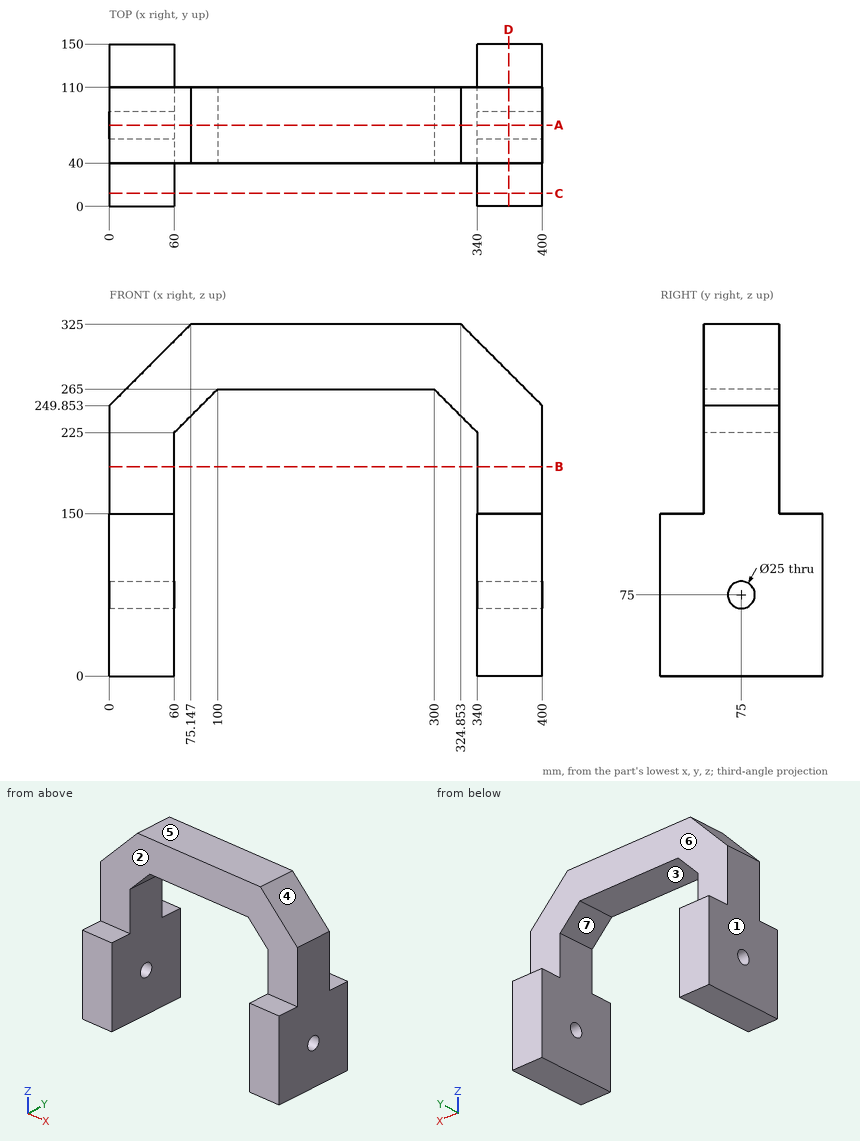
Here's the drawing with two shaded views (mm, measured from the low corner). I have some questions. A direction names the side the tool comes from. Coordinates: 2 decimals unless noted, no trailing zeros. Write each loop counter-clockwise with the first axis right and the second up, starting at its lowest first coordinate (ties: lowest second). Pieces come first, ordered by that corner, then holes. Notation, with made-up numbers: (17.5, 13.5) -> (22.5, 13.5) arc R36 ccw to (22.5, 52.5) -> close; hole circle Ø11 at (46.25, 13). An arc over 180 degrees is marked (long way). Write item = value, one per line. Start each with the question number.
(1) I want a section at B-B (z = 193.5). Please give me the cut outline in (x, y), plus the area to 3 significant figures.
(2) Which directions (+Z, -Z, +X, -X, +Y, -Y) give clear straight access to the entire face, cutting with the end or side of a thin tool? Please do the marked faces 5, 6 and 7.
(3) I want a section at C-C (y = 12). Please give me the cut outline in (x, z), plus the area to 3 significant figures.
(4) We'd pull the mould along X, two halves only. Please class the marked faces 1, 2, 3 and 4: released by +X, released by -X, zero draft, split by the parting line, or undercut.
(5) I want a section at A-A (y = 75). Please give me the cut outline in (x, z).
(6) Will these pins go through, and if not, where does the flat tip stop? pin 1 (12 mm diameter, centred on x = 18.5, y = 24, fed in from +Z); pin 2 (5 mm diameter, centred on x = 80.5, y = 76, fed in from -Z); pin 3 (12 mm diameter, centred on x = 199, y = 100, fed in from -Z).
(7) I need wall thicknesses on line 1 (X direction, y = 17, z = 122); line 2 (Y direction, x = 31, z = 245); line 3 (Z direction, x = 361, y = 111). Which ranges of each line are inside material? Lowest first, please. Write a range as [from, to].
(8) I want a section at D-D (x = 369). Please give me the cut outline in (y, z), plus the area to 3 significant figures.
Result set:
q1.outline = (0, 40) -> (60, 40) -> (60, 110) -> (0, 110) -> close; (340, 40) -> (400, 40) -> (400, 110) -> (340, 110) -> close
q1.area = 8,400 mm2
q2.face_5 = +Z, +X, -X, +Y, -Y
q2.face_6 = +Z, +X, -X, +Y
q2.face_7 = -Z, +Y, -Y
q3.outline = (0, 0) -> (60, 0) -> (60, 150) -> (0, 150) -> close; (340, 0) -> (400, 0) -> (400, 150) -> (340, 150) -> close
q3.area = 18,000 mm2
q4.face_1 = released by -X
q4.face_2 = zero draft
q4.face_3 = undercut
q4.face_4 = released by +X
q5.outline = (0, 0) -> (60, 0) -> (60, 62.5) -> (0, 62.5) -> close; (0, 87.5) -> (60, 87.5) -> (60, 225) -> (100, 265) -> (300, 265) -> (340, 225) -> (340, 87.5) -> (400, 87.5) -> (400, 249.85) -> (324.85, 325) -> (75.15, 325) -> (0, 249.85) -> close; (340, 0) -> (400, 0) -> (400, 62.5) -> (340, 62.5) -> close
q6.pin_1 = 150
q6.pin_2 = 243
q6.pin_3 = 265
q7.line_1 = [0, 60], [340, 400]
q7.line_2 = [40, 110]
q7.line_3 = [0, 150]
q8.outline = (0, 0) -> (150, 0) -> (150, 150) -> (110, 150) -> (110, 280.85) -> (40, 280.85) -> (40, 150) -> (0, 150) -> close; hole circle Ø25 at (75, 75)
q8.area = 31,200 mm2
